from build123d import *

# Parameters (mm, degrees)
SKETCH1_R                = 100
BOSS_EXTRUDE1_DEPTH      = 100
BOSS_EXTRUDE2_DEPTH      = 20
BOSS_EXTRUDE2_DEPTH_BACK = 20
SKETCH2_W                = 25
SKETCH2_H                = 10
SKETCH4_R                = 5
CUT_EXTRUDE1_DEPTH       = 20


with BuildPart() as part:
    # Sketch1 → Boss-Extrude1 (new body)
    with BuildSketch(Plane.XY):
        Circle(SKETCH1_R)
    extrude(amount=BOSS_EXTRUDE1_DEPTH)

    # Sketch2 → Boss-Extrude2 (add, two sides: drawn at the far end of the back side and taken through both)
    with BuildSketch(Plane(origin=(0, 0, 0), x_dir=(-1, 0, 0), z_dir=(0, 0, -1)).offset(-BOSS_EXTRUDE2_DEPTH_BACK)):
        Rectangle(SKETCH2_W, SKETCH2_H)
    extrude(amount=BOSS_EXTRUDE2_DEPTH + BOSS_EXTRUDE2_DEPTH_BACK)

    # Sketch4 → Cut-Extrude1 (cut)
    with BuildSketch(Plane.XZ.offset(5)):
        with Locations(Location((0, -10, 0), (0, 0, 270))):
            Circle(SKETCH4_R)
    extrude(amount=-CUT_EXTRUDE1_DEPTH, mode=Mode.SUBTRACT)


solid = part.part
Read the model definition and answer for the solid it produces. Units are mm, in the model's axes. A direction names the side the tool comes from. Give positions to 0.01 mm unless a question says otherwise; leave off trailing zeros. Loops run counter-clockwise (first coordinate to the right, second up) from the corner with the lowest first, then second, coordinate; pieces in that order, holes last. Notation, with made-up numbers: (-35.5, -30.75) -> (10.5, -30.75) arc R18 cw to (10.5, -1.75) -> close; hole circle Ø6 at (55, 23). An arc over 180 degrees is marked (long way). Answer as CSV lines item,"result".
Item 1: Find section B-B on y = 0. Give the vertices of the cut face in (x, z), plus the area to 3 significant figures.
Returned:
outline,"(-100, 0) -> (-12.5, 0) -> (-12.5, -20) -> (12.5, -20) -> (12.5, 0) -> (100, 0) -> (100, 100) -> (-100, 100) -> close; hole circle Ø10 at (0, -10)"
area,"20,400 mm²"
Item 2: Find section A-A on x = 0. Give the vertices of the cut face in (y, z).
Returned:
outline,"(-100, 0) -> (-5, 0) -> (-5, -5) -> (5, -5) -> (5, 0) -> (100, 0) -> (100, 100) -> (-100, 100) -> close; (-5, -20) -> (5, -20) -> (5, -15) -> (-5, -15) -> close"
Item 3: Find section C-C on z = -10. Give the vertices of the cut face in (x, y).
Returned:
outline,"(-12.5, -5) -> (-5, -5) -> (-5, 5) -> (-12.5, 5) -> close; (5, -5) -> (12.5, -5) -> (12.5, 5) -> (5, 5) -> close"
Item 4: Each of these flat-tipped pins is pushed along its axis until it touches: pin 1 (5 mm diameter, centred on x = 64.5, y = 77.5, fed in from -Z); pin 2 (1.5 mm diameter, centred on y = -61.5, z = 35, fed in from -X); pin 3 (16 mm diameter, centred on x = 5.5, z = -13, fed in from +Y). Where does it stop, or does it pass through?
Returned:
pin 1,"stops at z = 0"
pin 2,"stops at x = -79.43"
pin 3,"stops at y = 5"
Item 5: For faces 1 (the face through (3, 5, -5)), 2 (the face through (-12.5, 0, -10)), 3 (the face through (3, -5, -5)), determine the directions among +Z, -Z, +X, -X, +Y, -Y from which every point of the face is accessible in a straight line to the end or side of a thin tool.
Returned:
face 1,"-Z, +X, -X, +Y"
face 2,"-Z, -X, +Y, -Y"
face 3,"-Z, +X, -X, -Y"
Item 6: Determine the mould class of faces 4 (the face through (1.5, -0.07, -14.77)), 5 (the face through (0, 0, -20)), 6 (the face through (12.5, 0, -10)) for opening direction Z: +Z half, -Z half, draft (parallel to the pull), parting line (faces both ways), or undercut.
Returned:
face 4,"undercut"
face 5,"-Z half"
face 6,"draft"
Item 7: Consider line 1 (X direction, y = 0.25, z = -10); line 2 (Y direction, x = 3, z = 70); line 3 (Y direction, x = 2, z = 54.5). Determine where each line is inside the solid, lowest interval first. Write a range as [from, to].
Returned:
line 1,"x = [-12.5, -5], [5, 12.5]"
line 2,"y = [-99.95, 99.95]"
line 3,"y = [-99.98, 99.98]"
Item 8: Find section D-D on z = 64.5. Give the vertices of the cut face in (x, y), plus the area to 3 significant figures.
Returned:
outline,"circle Ø200 at (0, 0)"
area,"31,400 mm²"
